Geometry: final body of the model. Coordinates: model frame, mm. Face numbers are marked on the shaded views. A direction names the side the tool comes from. Give positions to 0.01 mm unless a question says otherwise; leave off trailing zeros. Loops run counter-clockwise (first coordinate to the right, second up) from the corner with the lowest first, then second, coordinate; pieces in that order, holes last. Notation, with made-up numbers: (6.5, 13) -> (44.5, 13) arc R25 ccw to (44.5, 43) -> close; hole circle Ø7 at (50, -1). An arc over 180 degrees is marked (long way). Answer in a Markdown table with one row per item. Add a question column.
1) First-contact query: P1, Ø2.5, axis at y = 11.5, z = -9, coming from the +X side; P2, Ø1.5, axis at x = -20.5, y = 17, coming from the +Z side; P3, Ø0.5, axis at y = 8.5, z = -8, coming from the -X side; P4, Ø7.5, axis at y = 6, z = -9.5, coming from the -X side. Flat tips, straight axial feed; report the tip coordinate or a pass-through.
2) Section query D-D (z = -2.25). Return the cut outline in (x, y), plus the area to 3 significant figures.
3) Access query for the marked faces 4, 5 and 6. Directions: +Z, -Z, +X, -X, +Y, -Y. A direction counts if a zero-diameter tool reaches every point of the face in a straight line with its end or side. Return the directions, or none.
4) Draft query along X for the marked faces 1, 2 and 3. Return one class per face: +X half, -X half, draft (parallel to the pull), parting line (faces both ways), or undercut.
5) Section query B-B (x = -7.5). Return the cut outline in (y, z).
6) Line query: line 1 (Y direction, x = -8, z = -7.75); line 2 (X direction, y = 9.5, z = -7); line 3 (Z direction, x = -9, y = 17). Output: solid intervals per line, ascending. Write a range as from..to.
7) Section query C-C (y = 17). Return the cut outline in (x, z), plus the area to 3 significant figures.
8) Section query A-A (y = 6). Return the cut outline in (x, z), plus the area to 3 significant figures.
```python
from build123d import *

# Parameters (mm, degrees)
SALIENTE_EXTRUIR1_DEPTH = 20
CROQUIS4_W              = 8
CROQUIS4_H              = 17
CORTAR_EXTRUIR2_DEPTH   = 5.5
CROQUIS4_4_W            = 1.5
CROQUIS4_4_H            = 17
CORTAR_EXTRUIR3_DEPTH   = 4.5
CORTAR_EXTRUIR4_REACH   = 9.5
SALIENTE_EXTRUIR3_REACH = 20.5
CROQUIS7_W              = 9.5
CROQUIS7_H              = 0.4


with BuildPart() as part:
    # Croquis1 → Saliente-Extruir1 (new body)
    with BuildSketch(Plane(origin=(0, 0, 0), x_dir=(1, 0, 0), z_dir=(0, 1, 0))):
        Polygon((-11.5, 13), (0, 13), (0, 0), (-49.748866803, 5.005022664), (-49.648766349, 6), (-1.5, 1.658480671), (-1.5, 6), (-11.5, 6), align=None)
    extrude(amount=SALIENTE_EXTRUIR1_DEPTH)

    # Croquis4 → Cortar-Extruir2 (cut)
    with BuildSketch(Plane(origin=(0, 0, -13), x_dir=(-1, 0, 0), z_dir=(0, 0, -1))):
        with Locations((5.5, 10)):
            Rectangle(CROQUIS4_W, CROQUIS4_H)
    extrude(amount=-CORTAR_EXTRUIR2_DEPTH, mode=Mode.SUBTRACT)

    # Croquis4_4 → Cortar-Extruir3 (cut)
    with BuildSketch(Plane(origin=(0, 0, -13), x_dir=(-1, 0, 0), z_dir=(0, 0, -1))):
        with Locations((0.75, 10)):
            Rectangle(CROQUIS4_4_W, CROQUIS4_4_H)
    extrude(amount=-CORTAR_EXTRUIR3_DEPTH, mode=Mode.SUBTRACT)

    # Croquis6 → Cortar-Extruir4 (cut, up to next)
    with BuildSketch(Plane(origin=(0, 0, -7.5), x_dir=(-1, 0, 0), z_dir=(0, 0, -1)), mode=Mode.PRIVATE) as cortar_extruir4_sk1:
        with BuildLine():
            Line((7, 15), (7, 5))
            ThreePointArc((7, 5), (5.5, 3.5), (4, 5))
            Line((4, 5), (4, 15))
            ThreePointArc((4, 15), (5.5, 16.5), (7, 15))
        make_face()
    cortar_extruir4_tool1 = extrude(cortar_extruir4_sk1.sketch, amount=-CORTAR_EXTRUIR4_REACH, mode=Mode.PRIVATE) & part.part
    add(cortar_extruir4_tool1.solids().sort_by_distance((-5.5, 10, -7.5))[0], mode=Mode.SUBTRACT)

    # Croquis7 → Saliente-Extruir3 (add, up to next)
    with BuildSketch(Plane(origin=(0, 1.5, 0), x_dir=(1, 0, 0), z_dir=(0, 1, 0)), mode=Mode.PRIVATE) as saliente_extruir3_sk1:
        with Locations((-4.75, 12.8)):
            Rectangle(CROQUIS7_W, CROQUIS7_H)
    saliente_extruir3_tool1 = extrude(saliente_extruir3_sk1.sketch, amount=SALIENTE_EXTRUIR3_REACH, mode=Mode.PRIVATE) - part.part
    add(saliente_extruir3_tool1.solids().sort_by_distance((-4.75, 1.5, -12.8))[0])


solid = part.part
```
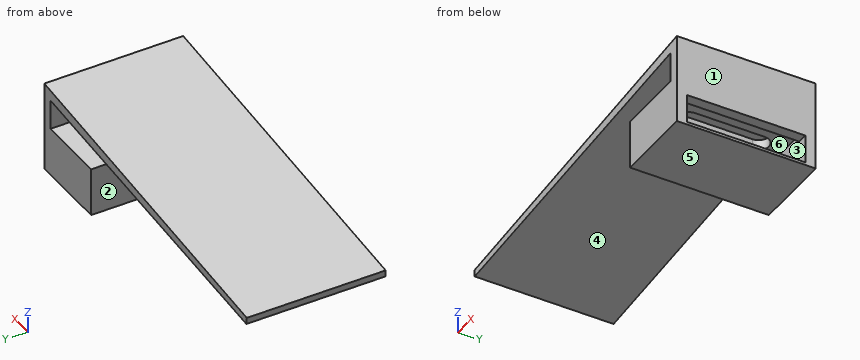
Evaluation:
| question | item | result |
|---|---|---|
| 1 | P1 | x = 0 |
| 1 | P2 | z = -1.99 |
| 1 | P3 | x = -11.5 |
| 1 | P4 | x = -49.67 |
| 2 | outline | (-22.36, 0) -> (-8.06, 0) -> (-8.06, 20) -> (-22.36, 20) -> close; (-1.5, 0) -> (0, 0) -> (0, 20) -> (-1.5, 20) -> close |
| 2 | area | 316 mm² |
| 3 | face 4 | +Y, -Y |
| 3 | face 5 | -Z, +X, -X, +Y, -Y |
| 3 | face 6 | none |
| 4 | face 1 | +X half |
| 4 | face 2 | -X half |
| 4 | face 3 | undercut |
| 5 | outline | (0, -13) -> (20, -13) -> (20, -6) -> (0, -6) -> close; (0, -2.2) -> (20, -2.2) -> (20, -0.75) -> (0, -0.75) -> close; hole (1.5, -12.6) -> (18.5, -12.6) -> (18.5, -7.5) -> (1.5, -7.5) -> close |
| 6 | line 1 | 0..1.5, 18.5..20 |
| 6 | line 2 | -11.5..-7, -4..0 |
| 6 | line 3 | -13..-12.6, -7.5..-6, -2.33..-0.91 |
| 7 | outline | (-49.75, -5.01) -> (-49.65, -6) -> (-1.5, -1.66) -> (-1.5, -6) -> (-11.5, -6) -> (-11.5, -13) -> (0, -13) -> (0, -12.6) -> (-9.5, -12.6) -> (-9.5, -7.5) -> (-1.5, -7.5) -> (-1.5, -8.5) -> (0, -8.5) -> (0, 0) -> close |
| 7 | area | 103 mm² |
| 8 | outline | (-49.75, -5.01) -> (-49.65, -6) -> (-1.5, -1.66) -> (-1.5, -6) -> (-4, -6) -> (-4, -7.5) -> (-1.5, -7.5) -> (-1.5, -8.5) -> (0, -8.5) -> (0, 0) -> close; (-11.5, -13) -> (0, -13) -> (0, -12.6) -> (-9.5, -12.6) -> (-9.5, -7.5) -> (-7, -7.5) -> (-7, -6) -> (-11.5, -6) -> close |
| 8 | area | 98.5 mm² |
